Work out the finished part from the listing and answer in its coordinate system (mm). Face numbers are marked on the shaded views. Coordinates: 2 decimals unless noted, no trailing zeros. Write each loop counter-clockwise with the first axis right and the second up, starting at its lowest first coordinate (ties: lowest second). Pieces come first, ordered by that corner, then holes. Notation, with made-up numbers: (2, -2.75) - (60, -2.75) arc R31 ccw to (60, 28.25) - close; hole circle Ø1 at (52.25, 41.5). An arc over 180 degrees is marked (long way). Answer as a JSON object with one key per item and string values. Group by question number.
from build123d import *

# Parameters (mm, degrees)
SKETCH1_W             = 40
SKETCH1_H             = 40
SKETCH1_R             = 14.5
BOSS_EXTRUDE1_DEPTH   = 40
M4_TAPPED_HOLE1_D     = 3.3
M4_TAPPED_HOLE1_DEPTH = 16.1
M4_TAPPED_HOLE1_TIP   = 0.991420021
M4_TAPPED_HOLE2_D     = 3.3
M4_TAPPED_HOLE2_DEPTH = 16.1
M4_TAPPED_HOLE2_TIP   = 0.991420021


with BuildPart() as part:
    # Sketch1 → Boss-Extrude1 (new body)
    with BuildSketch(Plane.XY):
        Rectangle(SKETCH1_W, SKETCH1_H)
        Circle(SKETCH1_R, mode=Mode.SUBTRACT)
    extrude(amount=BOSS_EXTRUDE1_DEPTH)

    # M4 Tapped Hole1
    with Locations(Plane(origin=(-13.435028843, 13.435028843, 40), x_dir=(1, 0, 0), z_dir=(0, 0, 1))):
        with Locations((0, 0), (26.870057686, 0), (26.870057686, -26.870057686), (0, -26.870057686)):
            Hole(M4_TAPPED_HOLE1_D / 2, depth=M4_TAPPED_HOLE1_DEPTH)
            with Locations((0, 0, -(M4_TAPPED_HOLE1_DEPTH + M4_TAPPED_HOLE1_TIP / 2))):  # 118° drill point
                Cone(0, M4_TAPPED_HOLE1_D / 2, M4_TAPPED_HOLE1_TIP, mode=Mode.SUBTRACT)

    # M4 Tapped Hole2
    with Locations(Plane(origin=(-10, -20, 30), x_dir=(-1, 0, 0), z_dir=(0, -1, 0))):
        with Locations((0, 0), (-20, 0), (-20, 20), (0, 20)):
            Hole(M4_TAPPED_HOLE2_D / 2, depth=M4_TAPPED_HOLE2_DEPTH)
            with Locations((0, 0, -(M4_TAPPED_HOLE2_DEPTH + M4_TAPPED_HOLE2_TIP / 2))):  # 118° drill point
                Cone(0, M4_TAPPED_HOLE2_D / 2, M4_TAPPED_HOLE2_TIP, mode=Mode.SUBTRACT)


solid = part.part
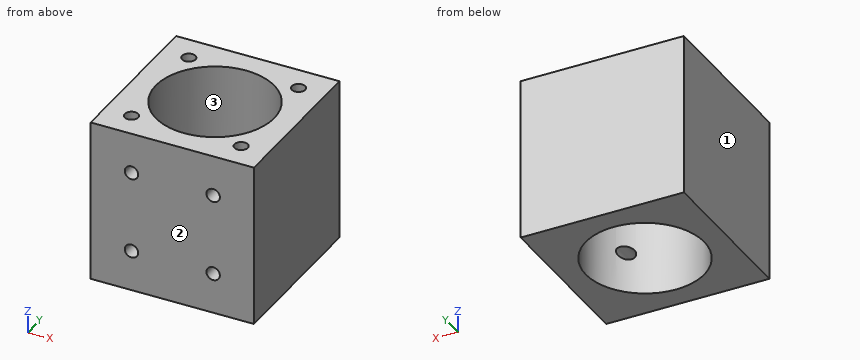
Q1. A flat-ended cylindrical pin translates along its axis: pin 1 Ø2.5 at (x, z) = (10, 30) entering from -Y. Find the tip coordinate at first contact, or state that the pin passes through.
Q2. Section C-C on z = 5.5 is taken. Determine the outline of the cut face in (x, y).
Q3. Section A-A on y = 0 is taken. Determine the outline of the cut face in (x, z).
Q4. Section B-B on x = 10 is taken. Determine the outline of the cut face in (y, z).
Q5. Consider L1, parallel to Z at x = -10, y = -11.25; L2, parallel to X at y = -17.25, z = 10; L3, parallel to Y at x = 6, z = 9. Determine where each line is inside the solid, lowest interval first. Write a range as from..to.
Q6. Section D-D on x = 6 is taken. Determine the outline of the cut face in (y, z), plus the area to 3 significant figures.
Q7. For a pull along X with two mould halves and no side action, classify the marked faces 1, 2 and 3 as +X half, -X half, draft (parallel to the pull), parting line (faces both ways), or undercut.
Numbers:
{
 "1": {"pin 1": "stops at y = 9.15"},
 "2": {"outline": "(-20, -20) - (20, -20) - (20, 20) - (-20, 20) - close; hole circle Ø29 at (0, 0)"},
 "3": {"outline": "(-20, 0) - (-14.5, 0) - (-14.5, 40) - (-20, 40) - close; (14.5, 0) - (20, 0) - (20, 40) - (14.5, 40) - close"},
 "4": {"outline": "(-20, 0) - (-10.5, 0) - (-10.5, 8.35) - (-20, 8.35) - close; (-20, 11.65) - (-10.5, 11.65) - (-10.5, 28.35) - (-20, 28.35) - close; (-20, 31.65) - (-10.5, 31.65) - (-10.5, 40) - (-20, 40) - close; (10.5, 0) - (20, 0) - (20, 40) - (10.5, 40) - close"},
 "5": {"L1": "z = 0..8.35, 11.65..28.35, 31.65..40", "L2": "x = -20..-11.65, -8.35..8.35, 11.65..20", "L3": "y = -20..-13.2, 13.2..20"},
 "6": {"outline": "(-20, 0) - (-13.2, 0) - (-13.2, 40) - (-20, 40) - close; (13.2, 0) - (20, 0) - (20, 40) - (13.2, 40) - close", "area": "544 mm²"},
 "7": {"face 1": "-X half", "face 2": "draft", "face 3": "undercut"}
}
